Autodesk Inventor part; units mm, degrees
ref_plane "РабПлоскость1" through (24.15, 22.2, 3) normal (1, 0, 0) x (0, 0, -1)
ref_plane "YZ Plane" through (0, 0, 0) normal (1, 0, 0) x (0, 1, 0)
ref_plane "XZ Plane" through (0, 0, 0) normal (0, 1, 0) x (-1, 0, 0)
sketch "Эскиз1" plane through (0, 0, 0) normal (0, 0, 1) x (1, 0, 0)
  line L0 (0, 0) -> (5, 0)
  line L1 (5, 0) -> (5, 18)
  line L2 (5, 18) -> (0, 18)
  line L3 (0, 18) -> (0, 0)
  line L4 (0, 0) -> (24.15, 0)
  line L5 (24.15, 0) -> (24.15, -5)
  line L6 (24.15, -5) -> (0, -5)
  line L7 (0, -5) -> (0, 0)
  dimension "d0" = 5
  dimension "d1" = 18
  dimension "d2" = 24.15
  dimension "d3" = 5
extrude "Выдавливание1" add sketch "Эскиз1" along normal blind 6
sketch "Эскиз4" plane through (0, 18, 0) normal (0, 1, 0) x (1, 0, 0)
  line L0 (0, 0) -> (0, -6)
  line L1 (0, 0) -> (0, -6)
  line L2 (5, 0) -> (0, 0)
  line L3 (0, 0) -> (0, -6)
  line L4 (5, -6) -> (0, -6)
  line L5 (5, 0) -> (5, -6)
extrude "Выдавливание2" add sketch "Эскиз4" along normal blind 7.2
fillet "Сопряжение1" radius 3 2 edges at (2.5, 25.2, 6) (2.5, 25.2, 0)
sketch "Эскиз5" plane through (5, 0, 6) normal (1, 0, 0) x (0, 0, -1)
  line L0 (0, -5) -> (0, -5)
  arc A0 (6, 22.2) -> (0, 22.2) centre (3, 22.2) ccw
  point P0 (6, 0)
  point P1 (6, -5)
  point P2 (2.5, 25.2)
hole "Отверстие2" at (5, 22.2, 3) direction (-1, 0, 0) diameter 3.2 depth 5
mirror "Зеркальное отражение1" about plane through (24.15, -5, 0) normal (1, 0, 0)
sketch "Эскиз9" plane through (0, 0, 0) normal (0, 0, -1) x (-1, 0, 0)
  line L0 (0, -5) -> (-48.3, -5)
  line L1 (-48.3, 22.2) -> (-48.3, -5)
  line L2 (-48.3, -5) -> (-45.3, -17.45)
  line L3 (-45.3, -17.45) -> (-45.3, -37.45)
  line L4 (-45.3, -37.45) -> (-37.3, -37.45)
  line L5 (-37.3, -37.45) -> (-37.3, -17.45)
  line L6 (-37.3, -17.45) -> (-40.3, -5)
  point P0 (0, 0)
  point P1 (-40.3, -5)
  dimension "d82" = 32.45
  dimension "d83" = 8
  dimension "d86" = 20
  dimension "d93" = 3
extrude "Выдавливание4" add sketch "Эскиз9" against normal blind 6
sketch "Эскиз11" plane through (0, 0, 6) normal (0, 0, 1) x (1, 0, 0)
  line L0 (41.3, -37.45) -> (41.3, -29.5)
  line L1 (37.3, -37.45) -> (45.3, -37.45)
  point P0 (0, 0)
  dimension "d91" = 7.95
hole "Отверстие6" at (41.3, -29.5, 6) direction (0, 0, -1) diameter 3.2 end through all
ref_plane "РабПлоскость1" through (24.15, 22.2, 3) normal (1, 0, 0) x (0, 0, -1)
mirror "Зеркальное отражение2" about plane through (24.15, 22.2, 3) normal (1, 0, 0) of "Выдавливание4", "Отверстие6"
fillet "Сопряжение3" radius 10 8 edges at (45.3, -17.45, 3) (37.3, -17.45, 3) (11, -17.45, 3) (3, -17.45, 3) (0, -5, 3) (8, -5, 3) (40.3, -5, 3) (48.3, -5, 3)
equation "\"Радиус_гибки\" = Толщина"
equation "\"Ширина_просечки\" = Толщина"
equation "\"Глубина_просечки\" = 0.5 * Толщина"
equation "\"Размер_просечки\" = 4 * Толщина"
equation "\"Мин_остаток\" = 2 * Толщина"
equation "\"Радиус_перехода\" = Радиус_гибки"
equation "\"Радиус_Якоби\" = Толщина"
equation "\"Размер_зазора\" = Толщина"
properties part number "Стойка для камеры"
Geometry check sheet. Reference: the model listing, model coordinates, mm. A direction names the side the tool comes from. Coordinates: 2 decimals unless noted, no trailing zeros. Order: outer loops, then holes, each group sorted by start corner. A loop starts at its lowest first (then second) coordinate and runs counter-clockwise, first axis right, second up. Notation, with made-up numbers: (70, 70) - (91, 70) arc R25 ccw to (91, 107) - close; hole circle Ø8 at (15, 17). An arc over 180 degrees is marked (long way). Answer as a JSON object with one key per item and string values. Group by question number.
Item 1: Scan lines: probe 1 along X at (y, z) = (-29.5, 1.35); probe 2 along X at (y, z) = (-27.5, 1.65); probe 3 along X at (y, z) = (19, 3.9). Record each from-to range of solid material in increasing order.
Item 2: Sectioned sample at A-A, the plane x = 41.3. Record the cut outline in (y, z).
Item 3: Depth check by flat-ended pin: pin 1 Ø1.8 at (x, z) = (24, 2) entering from -Y; pin 2 Ø2.5 at (x, y) = (7, -29.5) entering from +Z; pin 3 Ø1.5 at (y, z) = (-10.5, 0.5) entering from -X; pin 4 Ø1.8 at (y, z) = (-26.5, 3.5) entering from -X. Enter the tip coordinate at first touch or a pass-through.
Item 4: Draft check along Y on faces 4 (the face through (11, -28, 3)), 5 (the face through (24, 0, 3)), 6 (the face through (42.27, -28.23, 2.96)). Enter one of: +Y half, -Y half, draft (parallel to the pull), parting line (faces both ways), or undercut.
Item 5: Tool access check on faces 1 (the face through (5, 12, 3)), 2 (the face through (3, -28, 3)), 3 (the face through (37.3, -28, 3)). Record the directions out of +Z, -Z, +X, -X, +Y, -Y that give a thin tool (end or side, any length) a straight path to the whole face; none if there is none.
Item 6: Sectioned sample at C-C, the plane y = -29.5. Record the cut outline in (x, z).
Item 7: Sectioned sample at D-D, the plane y = -13. Record the cut outline in (x, z), and give its area (3 significant figures).
Item 8: Sectioned sample at B-B, the plane z = 2.2. Give the number of separate pieces and of enclosed holes in the cut face, and give its area (3 significant figures).
Resolved:
{
 "1": {"probe 1": "3 to 5.4, 8.6 to 11, 37.3 to 39.7, 42.9 to 45.3", "probe 2": "3 to 11, 37.3 to 45.3", "probe 3": "0 to 5, 43.3 to 48.3"},
 "2": {"outline": "(-37.45, 0) - (-31.1, 0) - (-31.1, 6) - (-37.45, 6) - close; (-27.9, 0) - (0, 0) - (0, 6) - (-27.9, 6) - close"},
 "3": {"pin 1": "y = -5", "pin 2": "through", "pin 3": "x = 1.14", "pin 4": "x = 3"},
 "4": {"face 4": "draft", "face 5": "+Y half", "face 6": "undercut"},
 "5": {"face 1": "+Z, -Z, +Y", "face 2": "+Z, -Z, -X, -Y", "face 3": "+Z, -Z, -Y"},
 "6": {"outline": "(3, 0) - (5.4, 0) - (5.4, 6) - (3, 6) - close; (8.6, 0) - (11, 0) - (11, 6) - (8.6, 6) - close; (37.3, 0) - (39.7, 0) - (39.7, 6) - (37.3, 6) - close; (42.9, 0) - (45.3, 0) - (45.3, 6) - (42.9, 6) - close"},
 "7": {"outline": "(1.93, 0) - (10.87, 0) - (10.87, 6) - (1.93, 6) - close; (37.43, 0) - (46.37, 0) - (46.37, 6) - (37.43, 6) - close", "area": "107 mm^2"},
 "8": {"separate pieces": "3", "enclosed holes": "2", "area": "1,040 mm^2"}
}
